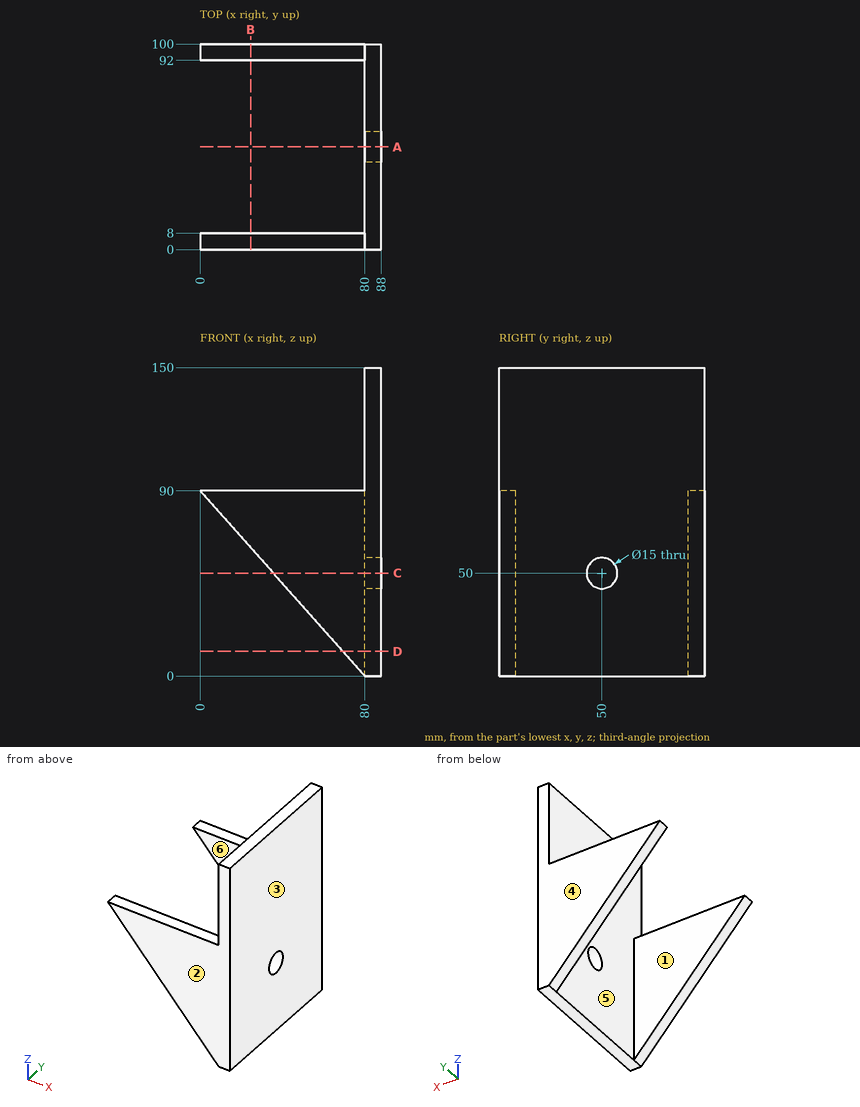
Could you check a few things on this drawing? It's one solid part, dimensions in mm from its lowest x, y, z. A direction names the side the tool comes from. Round coordinates to 2 decimals unless told otherwise and drop trailing zeros. Write each loop counter-clockwise with the first axis right and the second up, starting at its lowest first coordinate (ties: lowest second). Pieces come first, ordered by that corner, then holes. Notation, with made-up numbers: (14, 38.25) -> (41, 38.25) arc R17 ccw to (41, 69.25) -> close; hole circle Ø4 at (69, 52.5). An arc over 180 degrees is marked (long way). Use a Markdown table: item, result.
1. If we section it at A-A (y = 50): List the corners of the cut face in (x, z) for me.
Answer key:
| item | result |
|---|---|
| outline | (80, 0) -> (88, 0) -> (88, 42.5) -> (80, 42.5) -> close; (80, 57.5) -> (88, 57.5) -> (88, 150) -> (80, 150) -> close |
2. If we section it at C-C (z = 50): List the corners of the cut face in (x, y) for me, then the cut area to 3 significant figures.
Answer key:
| item | result |
|---|---|
| outline | (35.56, 0) -> (88, 0) -> (88, 42.5) -> (80, 42.5) -> (80, 8) -> (35.56, 8) -> close; (35.56, 92) -> (80, 92) -> (80, 57.5) -> (88, 57.5) -> (88, 100) -> (35.56, 100) -> close |
| area | 1,390 mm^2 |
3. Which directions (+Z, -Z, +X, -X, +Y, -Y) give clear straight access to the entire face, cutting with the end or side of a thin tool? Please do the marked faces 1 and 2.
Answer key:
| item | result |
|---|---|
| face 1 | +Z, -Z, -X |
| face 2 | +Z, -Z, +X, -X, -Y |
4. If we section it at B-B (x = 24.5): List the corners of the cut face in (y, z) for me.
Answer key:
| item | result |
|---|---|
| outline | (0, 62.44) -> (8, 62.44) -> (8, 90) -> (0, 90) -> close; (92, 62.44) -> (100, 62.44) -> (100, 90) -> (92, 90) -> close |
5. If we section it at D-D (z = 12): List the corners of the cut face in (x, y) for me, then the cut area to 3 significant figures.
Answer key:
| item | result |
|---|---|
| outline | (69.33, 0) -> (88, 0) -> (88, 100) -> (69.33, 100) -> (69.33, 92) -> (80, 92) -> (80, 8) -> (69.33, 8) -> close |
| area | 971 mm^2 |
6. For pin 1 Ø12 at (x, y) = (68.5, 18) entering from +Z; pin 2 Ø19.5 at (y, z) = (50, 50) entering from +X; pin 3 Ø5 at (y, z) = (33, 108) entering from -X; pin 4 Ø4 at (x, y) = (56, 95) entering from +Z, each with a flat end and sliding along its axis, tell me the tip position at first contact or that it passes through.
Answer key:
| item | result |
|---|---|
| pin 1 | passes through |
| pin 2 | stops at x = 88 |
| pin 3 | stops at x = 80 |
| pin 4 | stops at z = 90 |
7. Please list where these lines run through material, in increasing order: probe 1 along Y at (x, z) = (54, 35); probe 2 along Z at (x, y) = (82, 50); probe 3 along X at (y, z) = (41.5, 142).
Answer key:
| item | result |
|---|---|
| probe 1 | y = 0 to 8, 92 to 100 |
| probe 2 | z = 0 to 42.5, 57.5 to 150 |
| probe 3 | x = 80 to 88 |
8. We'd pull the mould along Y, two halves only. Please class the marked faces 3, 4, 5 and 6: +Y half, -Y half, draft (parallel to the pull), parting line (faces both ways), or undercut.
Answer key:
| item | result |
|---|---|
| face 3 | draft |
| face 4 | +Y half |
| face 5 | undercut |
| face 6 | undercut |
